Can you work these out from the model? Positions are in its coordinate system, mm. A direction names the side the tool comes from. Round coordinates to 2 decimals unless told otherwise and drop trailing zeros. Order: outer loops, then holes, each group sorted by start corner. A loop starts at its lowest first (then second) coordinate and runs counter-clockwise, first axis right, second up. Notation, with made-up numbers: M -30.75,22 L 25.25,22 A16 ccw 25.25,37 Z; hole C 30.5,56 d11. An arc over 180 degrees is marked long. Answer as a JSON object with one key per item and string values. Group by question number.
from build123d import *

# Parameters (mm, degrees)
SKETCH1_W             = 43
SKETCH1_H             = 48.1
SKETCH1_R             = 2.05
SKETCH1_R_2           = 6
BOSS_EXTRUDE1_DEPTH   = 12.5
SKETCH1_3_W           = 43
SKETCH1_3_H           = 10
BOSS_EXTRUDE2_DEPTH   = 3
MOVE_FACE1_BY         = 0.1
CROQUIS1_W            = 43
CROQUIS1_H            = 8.7
CORTAR_EXTRUIR1_DEPTH = 230.388992761
CROQUIS2_R            = 1.6
PINES_PRE_SERIE_DEPTH = 3
CROQUIS3_R            = 2.05
CORTAR_EXTRUIR2_DEPTH = 230.205824533


with BuildPart() as part:
    # Sketch1 → Boss-Extrude1 (new body)
    with BuildSketch(Plane.XY):
        with Locations((204, -15.05)):
            Rectangle(SKETCH1_W, SKETCH1_H)
        with Locations((217.423393759, -19.35)):
            Circle(SKETCH1_R, mode=Mode.SUBTRACT)
        with Locations((190.576606241, -34.85)):
            Circle(SKETCH1_R, mode=Mode.SUBTRACT)
        with Locations((217.423393759, -34.85)):
            Circle(SKETCH1_R, mode=Mode.SUBTRACT)
        with Locations((190.576606241, -19.35)):
            Circle(SKETCH1_R, mode=Mode.SUBTRACT)
        with Locations((204, -27.1)):
            Circle(SKETCH1_R_2, mode=Mode.SUBTRACT)
    extrude(amount=BOSS_EXTRUDE1_DEPTH)

    # Sketch1_3 → Boss-Extrude2 (add)
    with BuildSketch(Plane.XY):
        with Locations((204, 4)):
            Rectangle(SKETCH1_3_W, SKETCH1_3_H)
    extrude(amount=-BOSS_EXTRUDE2_DEPTH)

    # Move Face1: a face moved inward by 0.1
    extrude(part.faces().sort_by_distance((204, -1, -1.5))[0], amount=MOVE_FACE1_BY, dir=(0, 1, 0), mode=Mode.SUBTRACT)

    # Croquis1 → Cortar-Extruir1 (cut, through all)
    with BuildSketch(Plane(origin=(0, 0, -3), x_dir=(-1, 0, 0), z_dir=(0, 0, -1))):
        with Locations((-204, 4.65)):
            Rectangle(CROQUIS1_W, CROQUIS1_H)
    extrude(amount=-CORTAR_EXTRUIR1_DEPTH, mode=Mode.SUBTRACT)

    # Croquis2 → Pines Pre-serie (add)
    with BuildSketch(Plane(origin=(0, 0, 0), x_dir=(-1, 0, 0), z_dir=(0, 0, -1))):
        with Locations(Location((-210.9715045, -32.275, 0), (0, 0, 180))):
            Circle(CROQUIS2_R)
        with Locations(Location((-197.0284955, -32.275, 0), (0, 0, 180))):
            Circle(CROQUIS2_R)
    extrude(amount=PINES_PRE_SERIE_DEPTH)

    # Croquis3 → Cortar-Extruir2 (cut, through all)
    with BuildSketch(Plane(origin=(0, 0, 0), x_dir=(-1, 0, 0), z_dir=(0, 0, -1))):
        with Locations((-218.075, -27.1)):
            Circle(CROQUIS3_R)
        with Locations((-189.925, -27.1)):
            Circle(CROQUIS3_R)
    extrude(amount=-CORTAR_EXTRUIR2_DEPTH, mode=Mode.SUBTRACT)


solid = part.part
Item 1: If we mould it in two halves opening along Y, with no side actions, what happens to faces 1 (the face through (211, -32, -3)), 2 (the face through (219.379, -18.734, 6.162)), 3 (the face through (204, -39.1, 6))? For each: +Y half, -Y half, draft (parallel to the pull), parting line (faces both ways), or undercut.
Item 2: Suppose I cut it at A-A, the plane x = 204. Write out the boundary of the cut face in (y, z), and give its area (3 significant figures).
Item 3: I need wall thicknesses on line 1 (Y direction, x = 204, z = 10.25); line 2 (Y direction, x = 219, z = 10); line 3 (Y direction, x = 190.5, z = 8.5). Which ranges of each line are inside material? Lowest first, please.
Item 4: Suppose I cut it at B-B, the plane y = -34.85. Write out the boundary of the cut face in (x, z), and give its area (3 significant figures).
Item 5: On a 3-axis mill with a long thin cutter (end or side, diameter ignored), from which of +Z, -Z, +X, -X, +Y, -Y can I reach the whole of each face in a straight line? I mean faces 4 (the face through (198.506, -31.662, -1.479)), 5 (the face through (219.379, -34.234, 6.162)). Say none if no direction works.
Item 6: Suppose I cut it at C-C, the plane z = 1.75. Write out the boundary of the cut face in (x, y) (3 decimals).
Item 7: Suppose I cut it at D-D, the plane y = -16. Write out the boundary of the cut face in (x, z), and give its area (4 significant figures).
Item 8: I'm going to push flat-ended pins straight in: pin 1 Ø3.5 at (x, y) = (190.58, -34.85) entering from +Z; pin 2 Ø10 at (x, y) = (220, -6) entering from -Z. Where does each tip first touch, or does it pass through?
Computed:
{
 "1": {"face 1": "draft", "face 2": "undercut", "face 3": "-Y half"},
 "2": {"outline": "M -39.1,0 L -33.1,0 L -33.1,12.5 L -39.1,12.5 Z; M -21.1,0 L -0.9,0 L -0.9,-3 L 0.3,-3 L 0.3,12.5 L -21.1,12.5 Z", "area": "346 mm^2"},
 "3": {"line 1": "y = -39.1 to -33.1, -21.1 to 0.3", "line 2": "y = -39.1 to -36.16, -33.54 to -28.93, -25.27 to -20.66, -18.04 to 0.3", "line 3": "y = -39.1 to -36.9, -32.8 to -29.07, -25.13 to -21.4, -17.3 to 0.3"},
 "4": {"outline": "M 182.5,0 L 188.53,0 L 188.53,12.5 L 182.5,12.5 Z; M 192.63,0 L 215.37,0 L 215.37,12.5 L 192.63,12.5 Z; M 219.47,0 L 225.5,0 L 225.5,12.5 L 219.47,12.5 Z", "area": "435 mm^2"},
 "5": {"face 4": "-Z", "face 5": "+Z, -Z"},
 "6": {"outline": "M 182.5,-39.1 L 225.5,-39.1 L 225.5,0.3 L 182.5,0.3 Z; hole C 189.925,-27.1 d4.1; hole C 190.577,-34.85 d4.1; hole C 190.577,-19.35 d4.1; hole C 204,-27.1 d12; hole C 217.423,-34.85 d4.1; hole C 217.423,-19.35 d4.1; hole C 218.075,-27.1 d4.1"},
 "7": {"outline": "M 182.5,0 L 225.5,0 L 225.5,12.5 L 182.5,12.5 Z", "area": "537.5 mm^2"},
 "8": {"pin 1": "passes through", "pin 2": "stops at z = 0"}
}
